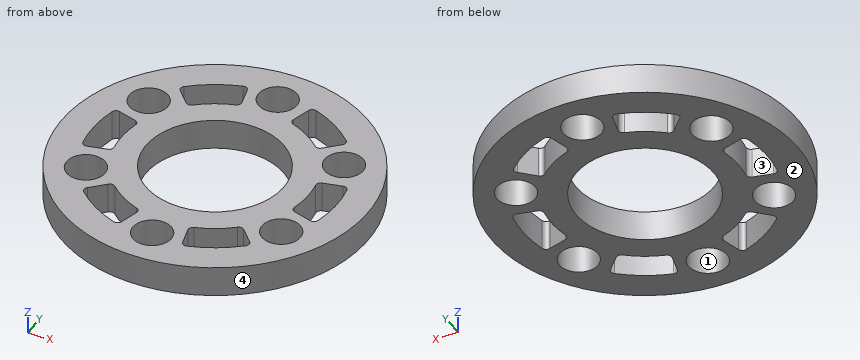
from build123d import *

# Parameters (mm, degrees)
F0_R     = 31.75
F0_R_2   = 4.0005
F0_R_3   = 14.3002
F1_DEPTH = 6.35


with BuildPart() as f1:
    # F0 (on Top) → F1 (new body)
    with BuildSketch(Plane.XY):
        Circle(F0_R)
        with BuildLine():
            ThreePointArc((-6.226129, -18.486919), (-5.669229, -18.957696), (-5.585454, -19.682094))
            Line((-5.585454, -19.682094), (-6.625875, -23.564999))
            ThreePointArc((-6.625875, -23.564999), (-7.110205, -24.179255), (-7.889173, -24.250619))
            ThreePointArc((-7.889173, -24.250619), (-12.886326, -22.006231), (-17.288853, -18.746391))
            ThreePointArc((-17.288853, -18.746391), (-17.607672, -18.038216), (-17.317734, -17.317734))
            Line((-17.317734, -17.317734), (-14.477198, -14.477198))
            ThreePointArc((-14.477198, -14.477198), (-13.800681, -14.187347), (-13.110948, -14.444165))
            ThreePointArc((-13.110948, -14.444165), (-9.877581, -16.821541), (-6.226129, -18.486919))
        make_face(mode=Mode.SUBTRACT)
        with Locations((-20.62223, -11.90625)):
            Circle(F0_R_2, mode=Mode.SUBTRACT)
        with Locations((0, -23.8125)):
            Circle(F0_R_2, mode=Mode.SUBTRACT)
        with BuildLine():
            ThreePointArc((12.897077, -14.635446), (13.583232, -14.388544), (14.252466, -14.678192))
            Line((14.252466, -14.678192), (17.094951, -17.520676))
            ThreePointArc((17.094951, -17.520676), (17.384746, -18.247246), (17.057066, -18.957534))
            ThreePointArc((17.057066, -18.957534), (12.614792, -22.163001), (7.590424, -24.345781))
            ThreePointArc((7.590424, -24.345781), (6.817717, -24.267799), (6.338731, -23.656465))
            Line((6.338731, -23.656465), (5.299022, -19.77622))
            ThreePointArc((5.299022, -19.77622), (5.386262, -19.045414), (5.95354, -18.576496))
            ThreePointArc((5.95354, -18.576496), (9.629092, -16.965006), (12.897077, -14.635446))
        make_face(mode=Mode.SUBTRACT)
        with Locations((20.62223, -11.90625)):
            Circle(F0_R_2, mode=Mode.SUBTRACT)
        with BuildLine():
            ThreePointArc((19.123206, 3.851473), (19.252461, 4.569152), (19.83792, 5.003902))
            Line((19.83792, 5.003902), (23.720826, 6.044323))
            ThreePointArc((23.720826, 6.044323), (24.494951, 5.932009), (24.946239, 5.293085))
            ThreePointArc((24.946239, 5.293085), (25.501118, -0.15677), (24.879277, -5.599391))
            ThreePointArc((24.879277, -5.599391), (24.425389, -6.229583), (23.656465, -6.338731))
            Line((23.656465, -6.338731), (19.77622, -5.299022))
            ThreePointArc((19.77622, -5.299022), (19.186944, -4.858067), (19.064488, -4.132331))
            ThreePointArc((19.064488, -4.132331), (19.506672, -0.143465), (19.123206, 3.851473))
        make_face(mode=Mode.SUBTRACT)
        with BuildLine():
            ThreePointArc((-19.123206, -3.851473), (-19.252461, -4.569152), (-19.83792, -5.003902))
            Line((-19.83792, -5.003902), (-23.720826, -6.044323))
            ThreePointArc((-23.720826, -6.044323), (-24.494951, -5.932009), (-24.946239, -5.293085))
            ThreePointArc((-24.946239, -5.293085), (-25.501118, 0.15677), (-24.879277, 5.599391))
            ThreePointArc((-24.879277, 5.599391), (-24.425389, 6.229583), (-23.656465, 6.338731))
            Line((-23.656465, 6.338731), (-19.77622, 5.299022))
            ThreePointArc((-19.77622, 5.299022), (-19.186944, 4.858067), (-19.064488, 4.132331))
            ThreePointArc((-19.064488, 4.132331), (-19.506672, 0.143465), (-19.123206, -3.851473))
        make_face(mode=Mode.SUBTRACT)
        with Locations((-20.62223, 11.90625)):
            Circle(F0_R_2, mode=Mode.SUBTRACT)
        with BuildLine():
            ThreePointArc((-12.897077, 14.635446), (-13.583232, 14.388544), (-14.252466, 14.678192))
            Line((-14.252466, 14.678192), (-17.094951, 17.520676))
            ThreePointArc((-17.094951, 17.520676), (-17.384746, 18.247246), (-17.057066, 18.957534))
            ThreePointArc((-17.057066, 18.957534), (-12.614792, 22.163001), (-7.590424, 24.345781))
            ThreePointArc((-7.590424, 24.345781), (-6.817717, 24.267799), (-6.338731, 23.656465))
            Line((-6.338731, 23.656465), (-5.299022, 19.77622))
            ThreePointArc((-5.299022, 19.77622), (-5.386262, 19.045414), (-5.95354, 18.576496))
            ThreePointArc((-5.95354, 18.576496), (-9.629092, 16.965006), (-12.897077, 14.635446))
        make_face(mode=Mode.SUBTRACT)
        Circle(F0_R_3, mode=Mode.SUBTRACT)
        with Locations((20.62223, 11.90625)):
            Circle(F0_R_2, mode=Mode.SUBTRACT)
        with BuildLine():
            Line((17.317734, 17.317734), (14.477198, 14.477198))
            ThreePointArc((14.477198, 14.477198), (13.800681, 14.187347), (13.110948, 14.444165))
            ThreePointArc((13.110948, 14.444165), (9.877581, 16.821541), (6.226129, 18.486919))
            ThreePointArc((6.226129, 18.486919), (5.669229, 18.957696), (5.585454, 19.682094))
            Line((5.585454, 19.682094), (6.625875, 23.564999))
            ThreePointArc((6.625875, 23.564999), (7.110205, 24.179255), (7.889173, 24.250619))
            ThreePointArc((7.889173, 24.250619), (12.886326, 22.006231), (17.288853, 18.746391))
            ThreePointArc((17.288853, 18.746391), (17.607672, 18.038216), (17.317734, 17.317734))
        make_face(mode=Mode.SUBTRACT)
        with Locations((0, 23.8125)):
            Circle(F0_R_2, mode=Mode.SUBTRACT)
    extrude(amount=F1_DEPTH)


solid = f1.part
The model under review builds one solid part; all positions refer to its coordinate system, in mm. Face numbers are marked on the shaded views. Round coordinates to 2 decimals unless told otherwise and drop trailing zeros. Order: outer loops, then holes, each group sorted by start corner. A loop starts at its lowest first (then second) coordinate and runs counter-clockwise, first axis right, second up. Notation, with made-up numbers: (-31, -4.75) -> (-18, -4.75) arc R31 cw to (-18, 25.25) -> close; hole circle Ø6 at (45, 51). An arc over 180 degrees is marked (long way). Use CSV: the item, a comma, the result in double quotes. Start each with the question number.
(1) Consider section D-D on x = 26.5. Write out the cut boundary in (y, z), and give its area (3 significant figures).
(2) Wall thickness on probe 1 along Y at (x, z) = (0, 2.25); probe 2 along X at (y, z) = (-9, 2.5); probe 3 along Y at (x, z) = (-2.5, 5.25): over which ranges is each line inside the solid? List them lowest first. Write a range as from..to.
(3) Consider section C-C on z = 1. State how many separate pieces and enclosed holes the cut face has, and give its area (3 significant figures).
(4) Consider section A-A on y = 0. Write out the cut boundary in (x, z).
(5) Mouldability with a two-part tool opening along X and no side actions: class the marked faces 1, 2, 3 and 4 as pulls with the +X half, pulls with the -X half, needs draft (parallel to the pull), parting line crosses it, or undercut.
(6) Consider section B-B on x = 0. Write out the cut boundary in (y, z).
(7) Insertion check: pin 1 (1 mm diameter, centred on x = 14, z = 4.5, fed in from +Y); pin 2 (1.5 mm diameter, centred on y = 15, z = 5.5, fed in from +X); pin 3 (2 mm diameter, centred on x = 3.5, z = 5.5, fed in from -Y). Each pin has a flat end and moves straight along its axis. Give the tip position at first contact, or say it passes through.
Responses:
1,outline,"(-17.49, 0) -> (17.49, 0) -> (17.49, 6.35) -> (-17.49, 6.35) -> close"
1,area,"222 mm²"
2,probe 1,"-31.75..-27.81, -19.81..-14.3, 14.3..19.81, 27.81..31.75"
2,probe 2,"-30.45..-23.37, -17.87..-11.11, 11.11..17.87, 23.37..30.45"
2,probe 3,"-31.65..-26.94, -20.69..-14.08, 14.08..20.69, 26.94..31.65"
3,separate pieces,"1"
3,enclosed holes,"13"
3,area,"1,810 mm²"
4,outline,"(-31.75, 0) -> (-25.5, 0) -> (-25.5, 6.35) -> (-31.75, 6.35) -> close; (-19.51, 0) -> (-14.3, 0) -> (-14.3, 6.35) -> (-19.51, 6.35) -> close; (14.3, 0) -> (19.51, 0) -> (19.51, 6.35) -> (14.3, 6.35) -> close; (25.5, 0) -> (31.75, 0) -> (31.75, 6.35) -> (25.5, 6.35) -> close"
5,face 1,"undercut"
5,face 2,"needs draft"
5,face 3,"undercut"
5,face 4,"parting line crosses it"
6,outline,"(-31.75, 0) -> (-27.81, 0) -> (-27.81, 6.35) -> (-31.75, 6.35) -> close; (-19.81, 0) -> (-14.3, 0) -> (-14.3, 6.35) -> (-19.81, 6.35) -> close; (14.3, 0) -> (19.81, 0) -> (19.81, 6.35) -> (14.3, 6.35) -> close; (27.81, 0) -> (31.75, 0) -> (31.75, 6.35) -> (27.81, 6.35) -> close"
7,pin 1,"y = 28.74"
7,pin 2,"x = 28.37"
7,pin 3,"y = -31.65"
